Here's how the part is built. I have some questions about the finished solid (model axes, mm). A direction names the side the tool comes from. Round coordinates to 2 decimals unless told otherwise and drop trailing zeros. Write each loop counter-clockwise with the first axis right and the second up, starting at its lowest first coordinate (ties: lowest second). Pieces come first, ordered by that corner, then holes. Notation, with made-up numbers: (9, 84) - (17, 84) arc R13 ccw to (17, 89) - close; hole circle Ø6 at (17, 89.25). An arc over 180 degrees is marked (long way). One line per question, with ' | ' between items. Start each with the question number.
(1) For faces 1 (the flat face through (9.75, 3, 53)), 2 (the flat face through (14, 1.5, 53)), 3 (the flat face through (18.75, 3, 53)), 4 (the flat face through (2.25, 2, 24)), which set-ups out of +Z, -Z, +X, -X, +Y, -Y let a thin tool reach every point of the face, with its end or its side?
(2) Imagine slicing it at A-A (z = 2). Write out the boundary of the cut face in (x, y).
(3) If I drill on L1, parallel to X at y = 1.1, z = 49.8; L2, parallel to X at y = -4.75, z = 40.5; L3, parallel to X at y = 1, z = 3, over which ranges is the centre line in solid material (lowest first)?
(4) Imagine slicing it at C-C (y = 1). Write out the boundary of the cut face in (x, z).
(5) Thinking about a two-plate mould opening in Z: for faces 5 (the flat face through (26.25, -5, 24)), 6 (the cylindrical face through (26.45, 0.74, 51.23)), 7 (the flat face through (27, -5, 4.757)), which applies, pulls with the +Z half, pulls with the -Z half, needs draft (parallel to the pull), parting line crosses it, or undercut?
(6) Will these pins go through, and if not, where does the flat tip stop? pin 1 (1.1 mm diameter, centred on x = 28, y = -4.5, fed in from -Z); pin 2 (8 mm diameter, centred on x = 4, z = 8.5, fed in from +Y); pin 3 (12 mm diameter, centred on x = 24.5, z = 34.5, fed in from -Y); pin 4 (1.1 mm diameter, centred on x = 1, z = 29, fed in from +Y).
(7) Imagine slicing it at D-D (x = 13.75). Write out the boundary of the cut face in (y, z).
(8) Imagine slicing it at B-B (y = -4). Write out the boundary of the cut face in (x, z).
from build123d import *

# Parameters (mm, degrees)
SKETCH_2_W      = 28.5
SKETCH_2_H      = 52
SKETCH_2_R      = 1.5
EXTRUDE_1_DEPTH = 1.5
EXTRUDE_2_DEPTH = 3
SKETCH_3_W      = 5.75
SKETCH_3_H      = 5.3
SKETCH_3_W_2    = 6.05
EXTRUDE_5_DEPTH = 3
SKETCH_5_W      = 19.2
SKETCH_5_H      = 39.7
EXTRUDE_6_DEPTH = 2
SKETCH_6_W      = 2.25
SKETCH_6_H      = 38.620640838
EXTRUDE_7_DEPTH = 1
SKETCH_6_3_W    = 2.25
SKETCH_6_3_H    = 38.620640838
EXTRUDE_8_DEPTH = 11.5


with BuildPart() as part:
    # Sketch 2 → Extrude 1 (new body)
    with BuildSketch(Plane(origin=(0, 0, 0), x_dir=(1, 0, 0), z_dir=(0, 1, 0))):
        with Locations((14.25, -26)):
            Rectangle(SKETCH_2_W, SKETCH_2_H)
        with Locations(Location((2.2, -2, 0), (0, 0, 270))):
            Circle(SKETCH_2_R, mode=Mode.SUBTRACT)
        with Locations(Location((26, -2, 0), (0, 0, 270))):
            Circle(SKETCH_2_R, mode=Mode.SUBTRACT)
        with Locations(Location((2.2, -49.8, 0), (0, 0, 90))):
            Circle(SKETCH_2_R, mode=Mode.SUBTRACT)
        with Locations(Location((26, -49.8, 0), (0, 0, 270))):
            Circle(SKETCH_2_R, mode=Mode.SUBTRACT)
    extrude(amount=EXTRUDE_1_DEPTH)

    # Sketch 1 → Extrude 2 (add)
    with BuildSketch(Plane(origin=(9.75, 1.5, 46.7), x_dir=(0.7893522173763263, 0, 0.6139406135149205), z_dir=(0, -1, 0))):
        Polygon((0, 0), (4.297584295, 5.525465522), (11.401754251, 0), (7.104169956, -5.525465522), align=None)
    extrude(amount=-EXTRUDE_2_DEPTH)

    # Sketch 3 → Extrude 5 (add)
    with BuildSketch(Plane(origin=(0, 1.5, 0), x_dir=(1, 0, 0), z_dir=(0, 1, 0))):
        with Locations((21.625, -49.35)):
            Rectangle(SKETCH_3_W, SKETCH_3_H)
        with Locations((6.725, -49.35)):
            Rectangle(SKETCH_3_W_2, SKETCH_3_H)
    extrude(amount=EXTRUDE_5_DEPTH)

    # Sketch 5 → Extrude 6 (add)
    with BuildSketch(Plane(origin=(0, 1.5, 0), x_dir=(1, 0, 0), z_dir=(0, 1, 0))):
        with Locations((14.25, -26.85)):
            Rectangle(SKETCH_5_W, SKETCH_5_H)
    extrude(amount=EXTRUDE_6_DEPTH)

    # Sketch 6 → Extrude 7 (add)
    with BuildSketch(Plane(origin=(0, 1.5, 0), x_dir=(1, 0, 0), z_dir=(0, 1, 0))):
        with Locations((27.375, -24.067488006)):
            Rectangle(SKETCH_6_W, SKETCH_6_H)
        with Locations((1.125, -24.067488006)):
            Rectangle(SKETCH_6_W, SKETCH_6_H)
    extrude(amount=EXTRUDE_7_DEPTH)

    # Sketch 6_3 → Extrude 8 (add)
    with BuildSketch(Plane(origin=(0, 1.5, 0), x_dir=(1, 0, 0), z_dir=(0, 1, 0))):
        with Locations((1.125, -24.067488006)):
            Rectangle(SKETCH_6_3_W, SKETCH_6_3_H)
        with Locations((27.375, -24.067488006)):
            Rectangle(SKETCH_6_3_W, SKETCH_6_3_H)
    extrude(amount=-EXTRUDE_8_DEPTH)


solid = part.part
Check sheet entries:
1) face 1: +Z, -X, +Y, -Y | face 2: +Z, +X, -X, -Y | face 3: +Z, +X, +Y, -Y | face 4: +Z, -Z, +Y
2) outline: (0, 0) - (0.7, 0) - (0.7, 1.5) - (0, 1.5) - close; (3.7, 0) - (24.5, 0) - (24.5, 1.5) - (3.7, 1.5) - close; (27.5, 0) - (28.5, 0) - (28.5, 1.5) - (27.5, 1.5) - close
3) L1: 0 to 0.7, 3.7 to 24.5, 27.5 to 28.5 | L2: 0 to 2.25, 26.25 to 28.5 | L3: 0 to 1.08, 3.32 to 24.88, 27.12 to 28.5
4) outline: (0, 0) - (28.5, 0) - (28.5, 52) - (0, 52) - close; hole circle Ø3 at (2.2, 2); hole circle Ø3 at (2.2, 49.8); hole circle Ø3 at (26, 2); hole circle Ø3 at (26, 49.8)
5) face 5: needs draft | face 6: undercut | face 7: pulls with the -Z half
6) pin 1: z = 4.76 | pin 2: y = 3.5 | pin 3: y = -10 | pin 4: y = 2.5
7) outline: (0, 0) - (1.5, 0) - (1.5, 7) - (3.5, 7) - (3.5, 46.7) - (4.5, 46.7) - (4.5, 53.7) - (1.5, 53.7) - (1.5, 52) - (0, 52) - close
8) outline: (0, 4.76) - (2.25, 4.76) - (2.25, 43.38) - (0, 43.38) - close; (26.25, 4.76) - (28.5, 4.76) - (28.5, 43.38) - (26.25, 43.38) - close
